Can you work these out from the model? Positions are in its coordinate system, mm. Face numbers are marked on the shaded views. A direction names the side the tool comes from. Round coordinates to 2 decimals unless told otherwise and drop trailing zeros. Order: outer loops, then holes, each group sorted by start corner. A loop starts at its lowest first (then second) coordinate and runs counter-clockwise, first axis right, second up. Notation, with made-up numbers: M -25,85.25 L 12,85.25 A7 cw 12,90.25 Z; hole C -4.5,6.5 d2. An arc over 180 degrees is marked long. Answer as a JSON object with one key per item and string values. Group by question number.
from build123d import *

# Parameters (mm, degrees)
SKETCH1_W           = 32.2
SKETCH1_H           = 25.5
BOSS_EXTRUDE1_DEPTH = 14.4
SKETCH3_W           = 32.2
SKETCH3_H           = 21.75
CUT_EXTRUDE1_DEPTH  = 12.4
SKETCH5_W           = 22.6
SKETCH5_H           = 2
CUT_EXTRUDE2_DEPTH  = 14.4
FILLET1_R           = 1
FILLET2_R           = 1
FILLET3_R           = 1
FILLET4_R           = 1
SKETCH10_R          = 1
CUT_EXTRUDE3_DEPTH  = 10
SKETCH11_W          = 4.85
SKETCH11_H          = 1.75
CUT_EXTRUDE4_DEPTH  = 20
FILLET5_R           = 1
SKETCH12_W          = 20
SKETCH12_H          = 2
BOSS_EXTRUDE2_DEPTH = 5
BOSS_EXTRUDE3_DEPTH = 5
SKETCH14_W          = 37.842545744
SKETCH14_H          = 22.134319208
CUT_EXTRUDE5_DEPTH  = 28.030214576
BOSS_EXTRUDE5_DEPTH = 3.75
CHAMFER1_SIZE       = 5
BOSS_EXTRUDE6_START = 1.5
SKETCH16_R          = 1
BOSS_EXTRUDE6_DEPTH = 1.5
SKETCH17_W          = 31.920460338
SKETCH17_H          = 22.260321026
CUT_EXTRUDE6_DEPTH  = 1


with BuildPart() as part:
    # Sketch1 → Boss-Extrude1 (new body)
    with BuildSketch(Plane.XY):
        Rectangle(SKETCH1_W, SKETCH1_H)
    extrude(amount=BOSS_EXTRUDE1_DEPTH)

    # Sketch3 → Cut-Extrude1 (cut)
    with BuildSketch(Plane.XY.offset(14.4)):
        with Locations((0, -0.125)):
            Rectangle(SKETCH3_W, SKETCH3_H)
    extrude(amount=-CUT_EXTRUDE1_DEPTH, mode=Mode.SUBTRACT)

    # Sketch5 → Cut-Extrude2 (cut)
    with BuildSketch(Plane.XY.offset(14.4)):
        with Locations((0, 11.75)):
            Rectangle(SKETCH5_W, SKETCH5_H)
    extrude(amount=-CUT_EXTRUDE2_DEPTH, mode=Mode.SUBTRACT)

    # Fillet1
    fillet1_edges = [part.edges().sort_by_distance(p)[0] for p in [
        (-11.3, 11.75, 14.4),
    ]]
    fillet(fillet1_edges, radius=FILLET1_R)

    # Fillet2
    fillet2_edges = [part.edges().sort_by_distance(p)[0] for p in [
        (-16.1, 11.75, 14.4),
    ]]
    fillet(fillet2_edges, radius=FILLET2_R)

    # Fillet3
    fillet3_edges = [part.edges().sort_by_distance(p)[0] for p in [
        (11.3, 11.75, 14.4),
    ]]
    fillet(fillet3_edges, radius=FILLET3_R)

    # Fillet4
    fillet4_edges = [part.edges().sort_by_distance(p)[0] for p in [
        (16.1, 11.75, 14.4),
    ]]
    fillet(fillet4_edges, radius=FILLET4_R)

    # Sketch10 → Cut-Extrude3 (cut)
    with BuildSketch(Plane(origin=(0, 12.75, 0), x_dir=(1, 0, 0), z_dir=(0, 1, 0))):
        with Locations(Location((-13.86, -8.203047487, 0), (0, 0, 270))):
            Circle(SKETCH10_R)
    cut_extrude3 = extrude(amount=-CUT_EXTRUDE3_DEPTH, mode=Mode.SUBTRACT)

    # Mirror1: Cut-Extrude3 across plane
    add(cut_extrude3.mirror(Plane(origin=(0, 0, 0), x_dir=(0, 0, 1), z_dir=(1, 0, 0))), mode=Mode.SUBTRACT)

    # Sketch11 → Cut-Extrude4 (cut)
    with BuildSketch(Plane.XY.offset(14.4)):
        with Locations((-13.675, -11.875)):
            Rectangle(SKETCH11_W, SKETCH11_H)
    cut_extrude4 = extrude(amount=-CUT_EXTRUDE4_DEPTH, mode=Mode.SUBTRACT)

    # Mirror2: Cut-Extrude4 across plane
    add(cut_extrude4.mirror(Plane(origin=(0, 0, 0), x_dir=(0, 0, 1), z_dir=(1, 0, 0))), mode=Mode.SUBTRACT)

    # Fillet5
    fillet5_edges = [part.edges().sort_by_distance(p)[0] for p in [
        (16.1, -11, 1),
        (11.25, -11.875, 14.4),
        (11.25, -11.875, 0),
        (-11.25, -11.875, 0),
        (-16.1, -11, 1),
        (-11.25, -11.875, 14.4),
    ]]
    fillet(fillet5_edges, radius=FILLET5_R)

    # Sketch12 → Boss-Extrude2 (add)
    with BuildSketch(Plane(origin=(0, 0, 0), x_dir=(-1, 0, 0), z_dir=(0, 0, -1))):
        with Locations((-2.6, 4.5)):
            Rectangle(SKETCH12_W, SKETCH12_H)
    extrude(amount=BOSS_EXTRUDE2_DEPTH)

    # Sketch13 → Boss-Extrude3 (add)
    with BuildSketch(Plane(origin=(0, 0, 0), x_dir=(-1, 0, 0), z_dir=(0, 0, -1))):
        Polygon((-12.6, 9), (7.4, 9), (7.4, 7), (7.4, 5.5), (6.4, 5.5), (6.4, 7), (-11.6, 7), (-11.6, 5.5), (-12.6, 5.5), (-12.6, 7), align=None)
    extrude(amount=BOSS_EXTRUDE3_DEPTH)

    # Sketch14 → Cut-Extrude5 (cut, through all)
    with BuildSketch(Plane.XZ.offset(-3.5)):
        with Locations((-0.315004543, 4.826001817)):
            Rectangle(SKETCH14_W, SKETCH14_H)
    extrude(amount=CUT_EXTRUDE5_DEPTH, mode=Mode.SUBTRACT)

    # Sketch15 → Boss-Extrude5 (add)
    with BuildSketch(Plane(origin=(0, 12.75, 0), x_dir=(1, 0, 0), z_dir=(0, 1, 0))):
        Polygon((11.3, 0), (12.6, 0), (12.6, 5), (-7.4, 5), (-7.4, 0), (-11.3, 0), (-11.3, -2), (11.3, -2), align=None)
    extrude(amount=-BOSS_EXTRUDE5_DEPTH)

    # Chamfer1
    # the kernel refuses this chamfer: 5 mm, written as the material it adds along each edge
    with BuildSketch(Plane(origin=(-7.4, 3.5, 0), x_dir=(-0.9996219169112968, 0, 0.027495876610586372), z_dir=(0, 1, 0))) as chamfer1_piece_1_section:
        Polygon((CHAMFER1_SIZE * 0.999621916911, -CHAMFER1_SIZE * 0.0274958766106), (-CHAMFER1_SIZE * 0.0274958766106, -CHAMFER1_SIZE * 0.999621916911), (0, 0), align=None)
    chamfer1_piece_1 = extrude(amount=9.25, mode=Mode.PRIVATE)
    chamfer1_piece_1 = split(chamfer1_piece_1, bisect_by=Plane(origin=(-9.052020772, 8.125, -5), z_dir=(0, 0, 1)), keep=Keep.TOP, mode=Mode.PRIVATE)
    add(chamfer1_piece_1)
    with BuildSketch(Plane(origin=(12.6, 3.5, 0), x_dir=(-0.027495876610586317, 0, -0.9996219169112968), z_dir=(0, 1, 0))) as chamfer1_piece_2_section:
        Polygon((CHAMFER1_SIZE * 0.999621916911, -CHAMFER1_SIZE * 0.0274958766106), (-CHAMFER1_SIZE * 0.0274958766106, -CHAMFER1_SIZE * 0.999621916911), (0, 0), align=None)
    chamfer1_piece_2 = extrude(amount=9.25, mode=Mode.PRIVATE)
    chamfer1_piece_2 = split(chamfer1_piece_2, bisect_by=Plane(origin=(16.1, 8.125, -1.788652221), z_dir=(-1, 0, 0)), keep=Keep.TOP, mode=Mode.PRIVATE)
    chamfer1_piece_2 = split(chamfer1_piece_2, bisect_by=Plane(origin=(13.973224067, 8.125, -5), z_dir=(0, 0, 1)), keep=Keep.TOP, mode=Mode.PRIVATE)
    add(chamfer1_piece_2)

    # Sketch16 → Boss-Extrude6 (add)
    with BuildSketch(Plane(origin=(0, 12.75, 0), x_dir=(1, 0, 0), z_dir=(0, 1, 0)).offset(BOSS_EXTRUDE6_START)):
        with BuildLine():
            Line((16.1, -13.4), (16.1, 1.5))
            Line((16.1, 1.5), (12.6, 5))
            Line((12.6, 5), (-7.4, 5))
            Line((-7.4, 5), (-12.4, 0))
            Line((-12.4, 0), (-16.1, 0))
            Line((-16.1, 0), (-16.1, -13.4))
            ThreePointArc((-16.1, -13.4), (-15.807106781, -14.107106781), (-15.1, -14.4))
            Line((-15.1, -14.4), (-12.3, -14.4))
            ThreePointArc((-12.3, -14.4), (-11.592893219, -14.107106781), (-11.3, -13.4))
            Line((-11.3, -13.4), (-11.3, -2))
            Line((-11.3, -2), (11.3, -2))
            Line((11.3, -2), (11.3, -13.4))
            ThreePointArc((11.3, -13.4), (11.592893219, -14.107106781), (12.3, -14.4))
            Line((12.3, -14.4), (15.1, -14.4))
            ThreePointArc((15.1, -14.4), (15.807106781, -14.107106781), (16.1, -13.4))
        make_face()
        with Locations(Location((13.86, -8.203047487, 0), (0, 0, 270))):
            Circle(SKETCH16_R, mode=Mode.SUBTRACT)
        with Locations(Location((-13.86, -8.203047487, 0), (0, 0, 270))):
            Circle(SKETCH16_R, mode=Mode.SUBTRACT)
    extrude(amount=-BOSS_EXTRUDE6_DEPTH)

    # Sketch17 → Cut-Extrude6 (cut)
    with BuildSketch(Plane(origin=(0, 0, -5), x_dir=(-1, 0, 0), z_dir=(0, 0, -1))):
        with Locations((-2.436035131, 9.274005754)):
            Rectangle(SKETCH17_W, SKETCH17_H)
    extrude(amount=-CUT_EXTRUDE6_DEPTH, mode=Mode.SUBTRACT)


solid = part.part
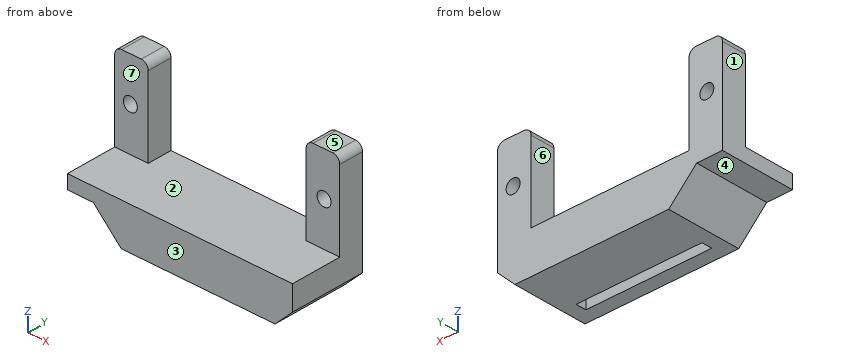
Item 1: Suppose I cut it at D-D, the plane z = 8.5. Write out the boundary of the cut face in (x, y).
Item 2: If we mould it in two halves opening along X, with no side actions, what happens to the marked faces 1, 2 and 3? For each: +X half, -X half, draft (parallel to the pull), parting line (faces both ways), or undercut.
Item 3: Suppose I cut it at B-B, the plane y = 6.25. Write out the boundary of the cut face in (x, z).
Item 4: I'm going to push flat-ended pins straight in: pin 1 Ø2 at (x, y) = (2, 9) entering from +Z; pin 2 Ø2 at (x, y) = (-12.5, 10.5) entering from -Z; pin 3 Ø2.5 at (x, z) = (13.86, 8.2) entering from -Y. Where does each tip first touch, or does it pass through?
Item 5: Suppose I cut it at C-C, the plane y = 12.75. Write out the boundary of the cut face in (x, z), and give its area (3 significant figures).
Item 6: I need wall thicknesses on line 1 (Z direction, x = 3.5, y = 7.5); line 2 (Y direction, x = 11.5, z = 11); line 3 (Z direction, x = -14, y = 6). Which ranges of each line are inside material? Lowest first, please.
Item 7: On a 3-axis mill with a long thin cutter (end or side, diameter ignored), from which of +Z, -Z, +X, -X, +Y, -Y can I reach the whole of each face in a straight line? I mean the marked faces 4, 5, 6 and 7. Say none if no direction works.
Item 8: Suppose I cut it at A-A, the plane x = -13.86. Write out the boundary of the cut face in (y, z), and give its area (3 significant figures).
Computed:
{
 "1": {"outline": "M -16.1,10.75 L -14.81,10.75 L -14.81,14.25 L -16.1,14.25 Z; M -12.91,10.75 L -11.3,10.75 L -11.3,14.25 L -12.91,14.25 Z; M 11.3,10.75 L 12.91,10.75 L 12.91,14.25 L 11.3,14.25 Z; M 14.81,10.75 L 16.1,10.75 L 16.1,14.25 L 14.81,14.25 Z"},
 "2": {"face 1": "-X half", "face 2": "undercut", "face 3": "draft"},
 "3": {"outline": "M -16.1,0 L -12.4,0 L -8.4,-4 L -6.4,-4 L -6.4,0 L 11.6,0 L 11.6,-4 L 13.6,-4 L 16.1,-1.5 L 16.1,2 L -16.1,2 Z"},
 "4": {"pin 1": "stops at z = 2", "pin 2": "stops at z = -0.9", "pin 3": "stops at y = 10.75"},
 "5": {"outline": "M -16.1,0 L -12.4,0 L -8.4,-4 L 13.6,-4 L 16.1,-1.5 L 16.1,13.4 A1 ccw 15.1,14.4 L 12.3,14.4 A1 ccw 11.3,13.4 L 11.3,2 L -11.3,2 L -11.3,13.4 A1 ccw -12.3,14.4 L -15.1,14.4 A1 ccw -16.1,13.4 Z; hole C -13.86,8.2 d2; hole C 13.86,8.2 d2", "area": "279 mm^2"},
 "6": {"line 1": "z = -4 to 2", "line 2": "y = 10.75 to 14.25", "line 3": "z = 0 to 2"},
 "7": {"face 4": "-Z, -X, +Y, -Y", "face 5": "+Z, +X, -X, +Y, -Y", "face 6": "+Z, +Y, -Y", "face 7": "+Z, +X, -X, -Y"},
 "8": {"outline": "M 3.5,0 L 14.25,0 L 14.25,7.2 L 10.75,7.2 L 10.75,2 L 3.5,2 Z; M 10.75,9.2 L 14.25,9.2 L 14.25,14.4 L 10.75,14.4 Z", "area": "57.9 mm^2"}
}
